Read the model definition and answer for the solid it produces. Units are mm, in the model's axes. A direction names the side the tool comes from. Give positions to 0.01 mm unless a question says otherwise; leave off trailing zeros. Loops run counter-clockwise (first coordinate to the right, second up) from the corner with the lowest first, then second, coordinate; pieces in that order, holes last. Notation, with made-up numbers: M 73.25,40.5 L 107.25,40.5 A20 ccw 107.25,55.5 Z; hole C -8.5,1 d3. An arc over 180 degrees is marked long. Return JSON: item names as keys, results as strings. Group by question number.
```python
from build123d import *

# Parameters (mm, degrees)
BASE_FLANGE1_START           = -6.35
BASE_FLANGE1_OUTLINE_W       = 19.05
BASE_FLANGE1_OUTLINE_H       = 19.05
BASE_FLANGE1_OUTLINE_R       = 3.175
BASE_FLANGE1_DEPTH           = 6.35
EDGE_FLANGE1_STRIP_W         = 26.8732
EDGE_FLANGE1_STRIP_H         = 6.35
EDGE_FLANGE1_STRIP_CUT_DEPTH = 19.05
EDGE_FLANGE1_DEPTH           = 19.05
SKETCH9_R                    = 8.73125
CUT_EXTRUDE1_DEPTH           = 36.497579143
FILLET2_R                    = 1.27


# Read off the part's stored shape, not the designer's step: Base-Flange1
# Sheet-metal steps are written as plain solids
with BuildPart() as part:
    # Base-Flange1 outline → Base-Flange1 (new body)
    with BuildSketch(Plane.XY.offset(BASE_FLANGE1_START)):
        Rectangle(BASE_FLANGE1_OUTLINE_W, BASE_FLANGE1_OUTLINE_H)
        with Locations((0, -3.175)):
            Circle(BASE_FLANGE1_OUTLINE_R, mode=Mode.SUBTRACT)
    extrude(amount=BASE_FLANGE1_DEPTH)

    # Edge-Flange1 strip (across the edge) → Edge-Flange1 strip cut (cut)
    with BuildSketch(Plane(origin=(9.525, 9.525, 0), x_dir=(0, -1, 0), z_dir=(-1, 0, 0))):
        with Locations((-6.35, -3.175)):
            Rectangle(EDGE_FLANGE1_STRIP_W, EDGE_FLANGE1_STRIP_H)
    extrude(amount=EDGE_FLANGE1_STRIP_CUT_DEPTH, mode=Mode.SUBTRACT)

    # Edge-Flange1 section (across the edge) → Edge-Flange1 (add)
    with BuildSketch(Plane(origin=(9.525, 9.525, 0), x_dir=(0, -1, 0), z_dir=(-1, 0, 0))):
        with BuildLine():
            Line((0, 0.7366), (0, 31.75))
            Line((0, 31.75), (6.35, 31.75))
            Line((6.35, 31.75), (6.35, 0.7366))
            ThreePointArc((6.35, 0.7366), (6.565745145, 0.215745145), (7.0866, 0))
            Line((7.0866, 0), (7.0866, -6.35))
            ThreePointArc((7.0866, -6.35), (2.075617084, -4.274382916), (0, 0.7366))
        make_face()
    extrude(amount=EDGE_FLANGE1_DEPTH)

    # Sketch9 → Cut-Extrude1 (cut, through all)
    with BuildSketch(Plane.XZ.offset(-3.175)):
        with Locations(Location((0, 16.2433, 0), (0, 0, 270))):
            Circle(SKETCH9_R)
    extrude(amount=-CUT_EXTRUDE1_DEPTH, mode=Mode.SUBTRACT)

    # Fillet2
    fillet2_edges = [part.edges().sort_by_distance(p)[0] for p in [
        (9.525, 6.35, 31.75),
        (-9.525, 6.35, 31.75),
        (9.525, -9.525, -3.175),
        (-9.525, -9.525, -3.175),
    ]]
    fillet(fillet2_edges, radius=FILLET2_R)


solid = part.part
```
1. Straight lines are drawn through the part: line 1 along Y through (x, z) = (0, -4.25) (3 decimals); line 2 along Y through (x, z) = (0, -1.5) (3 decimals); line 3 along Z through (x, y) = (-2, 7). For each, find the intervals that lie inside material, in ascending order.
2. Find section C-C (y = -1.25). Write down the section's boundary in (x, z) (3 decimals).
3. Find section B-B (z = 15.5). Write down the section's boundary in (x, y) (3 decimals).
4. For faces 5 (the flat face through (-2, -6, 0)), 6 (the flat face through (9.525, 4, 8)), determine the directions among +Z, -Z, +X, -X, +Y, -Y from which every point of the face is accessible in a straight line to the end or side of a thin tool.
5. The mould has two halves that part along Z. Classify faces 1 (the flat face through (-8.3, 3.175, 13)), 2 (the cylindrical face through (9.16, 6.31, 31.37)), 3 (the cylindrical face through (0.384, 6.306, 24.966)), 4 (the cylindrical face through (0.133, 7.394, -4.329)): +Z half, -Z half, draft (parallel to the pull), parting line (faces both ways), or undercut.
6. Flat-ended cylindrical pins translate along their axes: P1, Ø6, axis at x = 3.5, y = -5.5, coming from the +Z side; P2, Ø5.5, axis at x = -2, z = 22, coming from the -Y side (3 decimals). Find the tip coordinate at first contact, or state that the pin passes through.
7. Find section A-A (x = 0). Write down the section's boundary in (y, z) (3 decimals), and give its area (3 significant figures).
Result:
{
 "1": {"line 1": "y = -9.525 to -6.35, 0 to 7.474", "line 2": "y = -9.525 to -6.35, 0 to 9.163", "line 3": "z = -4.69 to 7.74, 24.74 to 31.75"},
 "2": {"outline": "M -9.525,-6.35 L -2.525,-6.35 L -2.525,0 L -9.525,0 Z; M 2.525,-6.35 L 9.525,-6.35 L 9.525,0 L 2.525,0 Z"},
 "3": {"outline": "M -9.525,3.175 L -8.7,3.175 L -8.7,9.525 L -9.525,9.525 Z; M 8.7,3.175 L 9.525,3.175 L 9.525,9.525 L 8.7,9.525 Z"},
 "4": {"face 5": "+Z, +X, -X, -Y", "face 6": "+Z, -Z, +X, +Y, -Y"},
 "5": {"face 1": "draft", "face 2": "+Z half", "face 3": "undercut", "face 4": "-Z half"},
 "6": {"P1": "stops at z = 0", "P2": "stops at y = 3.175"},
 "7": {"outline": "M -9.525,-6.35 L -6.35,-6.35 L -6.35,0 L -9.525,0 Z; M 0,-6.35 L 2.438,-6.35 A7.087 ccw 9.525,0.737 L 9.525,7.512 L 3.175,7.512 L 3.175,0.737 A0.737 cw 2.438,0 L 0,0 Z; M 3.175,24.975 L 9.525,24.975 L 9.525,31.75 L 3.175,31.75 Z", "area": "161 mm2"}
}
